The drawing under review shows one solid part. Ordinate dimensions are in mm from its lowest x, y, z. A direction names the side the tool comes from. Give positions to 0.01 mm unless a question says otherwise; leave off trailing zeros. Write each loop counter-clockwise with the first axis right and the second up, starting at its lowest first coordinate (ties: lowest second). Pieces come first, ordered by that corner, then holes. Notation, with made-up numbers: (83, 31.5) -> (93, 31.5) arc R5 cw to (93, 39.5) -> close; hole circle Ø8 at (-28.75, 29). An arc over 180 degrees is marked (long way). Put each result on its own line as item: value. Start each with the question number.
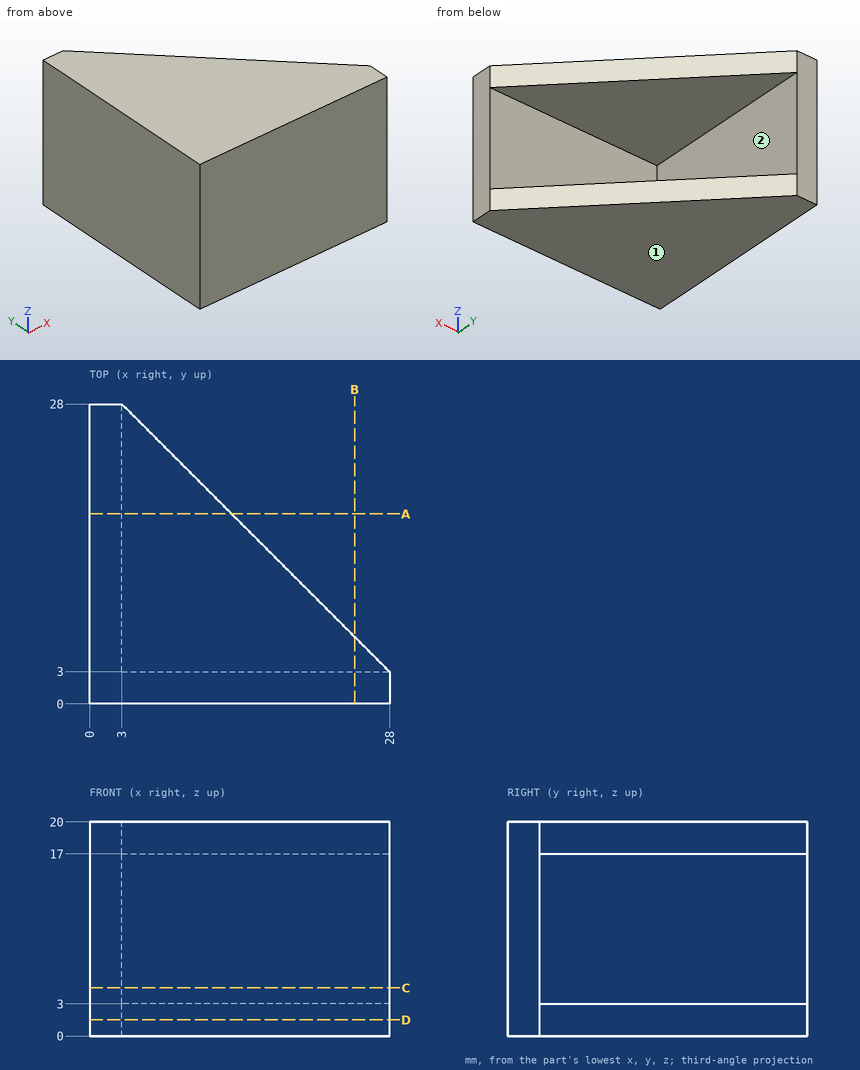
Q1. Take a section at A-A on y = 17.75. Give the boundary of the cut face in (x, z), then the cut area to 4 significant figures.
Q2. To check wall thickness, follow probe 1 along Z at (x, y) = (21, 4.5); probe 2 along Y at (x, z) = (7.25, 7). State the ranges of each line that lie inside material, in increasing order. Write a range as from..to.
Q3. Take a section at C-C on z = 4.5. Give the boundary of the cut face in (x, y).
Q4. Take a section at D-D on z = 1.5. Give the boundary of the cut face in (x, y).
Q5. For pin 1 (4 mm diameter, centred on y = 12.5, z = 17.5, fed in from +X); pin 2 (7 mm diameter, centred on y = 20, z = 8.5, fed in from +X); pin 3 (8 mm diameter, centred on x = 14.5, y = 20, fed in from +Z); pin 4 (5 mm diameter, centred on x = 21, z = 11.5, fed in from +Y), all flat-tipped, find the tip position at first contact; note any pin that passes through.
Q6. Take a section at B-B on x = 24.75. Give the boundary of the cut face in (y, z).
Q7. Machinability: for the marked faces 1 and 2, which of the approach directions +Z, -Z, +X, -X, +Y, -Y give a long, thin tool a straight path to every point of the face, cutting with its end or side? Answer none if there is none.
Result:
1. outline: (0, 0) -> (13.25, 0) -> (13.25, 3) -> (3, 3) -> (3, 17) -> (13.25, 17) -> (13.25, 20) -> (0, 20) -> close
1. area: 121.5 mm^2
2. probe 1: z = 0..3, 17..20
2. probe 2: y = 0..3
3. outline: (0, 0) -> (28, 0) -> (28, 3) -> (3, 3) -> (3, 28) -> (0, 28) -> close
4. outline: (0, 0) -> (28, 0) -> (28, 3) -> (3, 28) -> (0, 28) -> close
5. pin 1: stops at x = 20.5
5. pin 2: stops at x = 3
5. pin 3: stops at z = 20
5. pin 4: stops at y = 3
6. outline: (0, 0) -> (6.25, 0) -> (6.25, 3) -> (3, 3) -> (3, 17) -> (6.25, 17) -> (6.25, 20) -> (0, 20) -> close
7. face 1: -Z, +X, -X, +Y, -Y
7. face 2: +X, +Y
